Job drawing, mm, ordinate dimensions from the low corner. One solid piece. A direction names the side the tool comes from. Coordinates: 2 decimals unless noted, no trailing zeros. Write each loop counter-clockwise with the first axis right and the second up, starting at its lowest first coordinate (ties: lowest second). Pieces come first, ordered by that corner, then holes. Notation, with made-up numbers: (4.25, -39) -> (54.25, -39) arc R22 ccw to (54.25, -18) -> close; hole circle Ø5 at (54, 24). An arc over 180 degrees is marked (long way). One line per question, with ' | ' between items. Start each with the question number.
Item 1: 3-axis set-ups, long thin cutter, end or side, ignore diameter. For the marked faces 4, 5 and 6: which of +Z, -Z, +X, -X, +Y, -Y reach the whole face in a straight line?
Item 2: Saw through at C-C (x = 2). List the corners of the cut face in (y, z), and give its area (3 significant figures).
Item 3: Pin check, flat tips, straight feed: pin 1 (1.5 mm diameter, centred on x = 4.5, z = 11, fed in from +Y); pin 2 (5.5 mm diameter, centred on x = 2.5, y = 15, fed in from -Z); pin 3 (5 mm diameter, centred on x = 4.5, z = 2, fed in from -Y). Stop position of each tip, or through.
Item 4: Saw through at B-B (z = 13). List the corners of the cut face in (x, y).
Item 5: Saw through at A-A (y = 11). List the corners of the cut face in (x, z).
Item 6: Saw through at D-D (x = 4.5). List the corners of the cut face in (y, z).
Item 7: Probe probe 1 along Y at (x, z) = (6.75, 4); probe 2 along X at (y, z) = (7.5, 12.5); probe 3 along Z at (x, y) = (10, 2.4). List the from-to ranges inside material, lowest first. Write a range as [from, to].
Item 8: Two-plate mould, pull along X, no slides. Class the marked faces 1, 2 and 3: pulls with the +X half, pulls with the -X half, needs draft (parallel to the pull), parting line crosses it, or undercut.
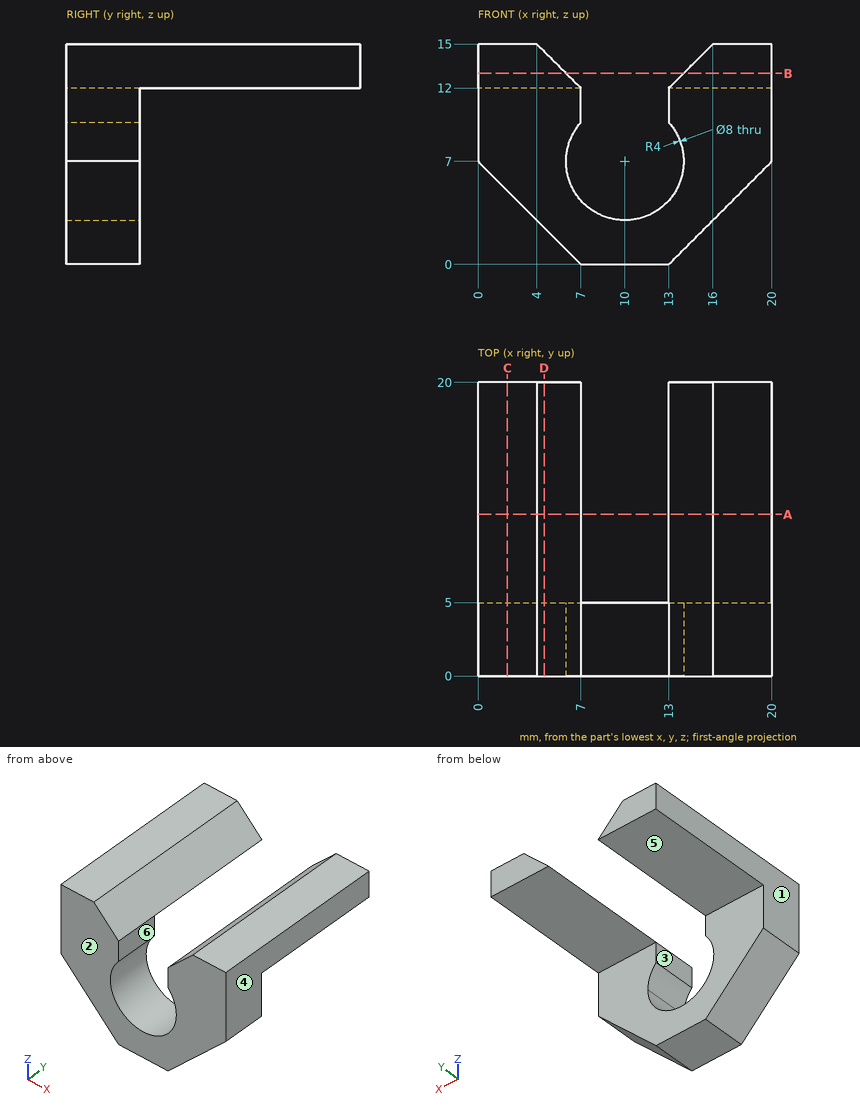
From the geometry:
1) face 4: +Z, -Z, +X, +Y, -Y | face 5: -Z, +X, -X, +Y | face 6: +Z, +Y, -Y
2) outline: (0, 5) -> (5, 5) -> (5, 12) -> (20, 12) -> (20, 15) -> (0, 15) -> close | area: 95.0 mm2
3) pin 1: y = 5 | pin 2: z = 12 | pin 3: y = 0
4) outline: (0, 0) -> (6, 0) -> (6, 20) -> (0, 20) -> close; (14, 0) -> (20, 0) -> (20, 20) -> (14, 20) -> close
5) outline: (0, 12) -> (7, 12) -> (4, 15) -> (0, 15) -> close; (13, 12) -> (20, 12) -> (20, 15) -> (16, 15) -> close
6) outline: (0, 2.5) -> (5, 2.5) -> (5, 12) -> (20, 12) -> (20, 14.5) -> (0, 14.5) -> close
7) probe 1: [0, 5] | probe 2: [0, 6.5], [13.5, 20] | probe 3: [0, 3]
8) face 1: pulls with the -X half | face 2: needs draft | face 3: undercut
